Input: part model. Units: mm. Frame: model coordinates. Face numbers are marked on the shaded views. Give positions to 0.01 mm unless a question says otherwise; leave off trailing zeros. Loops run counter-clockwise (first coordinate to the right, second up) from the corner with the lowest first, then second, coordinate; pieces in that order, holes last. Notation, with made-up numbers: M 25,26 L 73,26 A34 ccw 73,59 Z; hole C 61.25,24 d8. An arc over 180 degrees is marked long. Answer as a JSON object with one key per item and string values. Group by question number.
1) Ray query, L1, parallel to Z at x = 0, y = 3.75; L2, parallel to Z at x = 0, y = 6.5. Return the intervals inside material, ascending.
2) Section query B-B on y = 7.25. Return loops of the section in (x, z) (1 decimal), plus the area to 3 significant figures.
3) Draft query along Z for the marked faces 1, 2 and 3. Return one class per face: +Z half, -Z half, draft (parallel to the pull), parting line (faces both ways), or undercut.
4) Section query A-A on z = 0. Return loops of the section in (x, y).
5) Section query C-C on x = 0. Return loops of the section in (y, z).
6) Section query D-D on x = 7.5. Return loops of the section in (y, z).
7) First-contact query: P1, Ø2.5, axis at x = 0, z = 0, coming from the +Y side; P2, Ø6, axis at x = -6, z = 1.5, coming from the -Y side; P3, Ø1.5, axis at x = 5, y = 2, coming from the +Z side; P4, Ø1, axis at y = 6.5, z = -5.5, coming from the +X side. Flat tips, straight axial feed; report the tip coordinate or a pass-through.
Autodesk Inventor part; units mm, degrees
ref_plane "YZ Plane" through (0, 0, 0) normal (1, 0, 0) x (0, 1, 0)
ref_plane "XZ Plane" through (0, 0, 0) normal (0, 1, 0) x (-1, 0, 0)
ref_plane "XY Plane" through (0, 0, 0) normal (0, 0, 1) x (1, 0, 0)
sketch "Sketch1" plane through (0, 0, 0) normal (0, 1, 0) x (-1, 0, 0)
  circle A0 centre (0, 0) radius 13.081
  dimension "outerDiamKnurledKnob" = 26.162
extrude "Extrusion1" add sketch "Sketch1" along normal blind 4.064
sketch "Sketch2" plane through (0, 4.064, 0) normal (0, 1, 0) x (1, 0, 0)
  circle A0 centre (0, 0) radius 7.9375
  dimension "innerRingDiam" = 15.875
extrude "Extrusion2" add sketch "Sketch2" along normal blind 3.937
sketch "Sketch3" plane through (0, 8.001, 0) normal (0, 1, 0) x (1, 0, 0)
  point P0 (0, 0)
  point P1 (0, 0)
hole "Hole1" at (0, 8.001, 0) direction (0, -1, 0) diameter 3.9624 depth 6.35
properties part number "knurledKnob" material "Aluminum 6061"
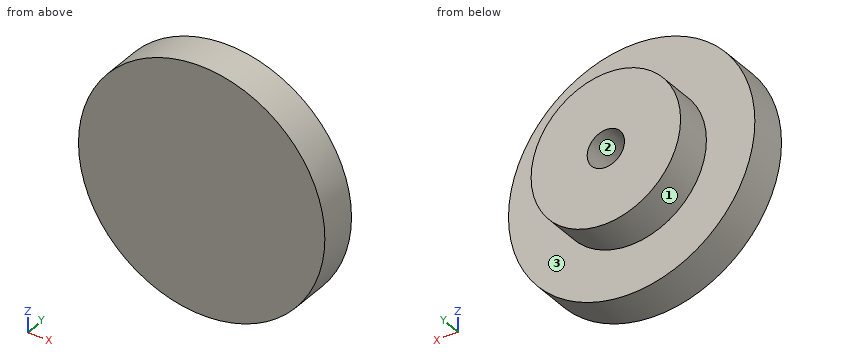
Output:
{
 "1": {"L1": "z = -13.08 to -1.98, 1.98 to 13.08", "L2": "z = -7.94 to -1.98, 1.98 to 7.94"},
 "2": {"outline": "C 0,0 d15.9; hole C 0,0 d4", "area": "186 mm^2"},
 "3": {"face 1": "parting line", "face 2": "undercut", "face 3": "draft"},
 "4": {"outline": "M -13.08,0 L 13.08,0 L 13.08,4.06 L 7.94,4.06 L 7.94,8 L 1.98,8 L 1.98,1.65 L -1.98,1.65 L -1.98,8 L -7.94,8 L -7.94,4.06 L -13.08,4.06 Z"},
 "5": {"outline": "M 0,-13.08 L 4.06,-13.08 L 4.06,-7.94 L 8,-7.94 L 8,-1.98 L 1.65,-1.98 L 1.65,1.98 L 8,1.98 L 8,7.94 L 4.06,7.94 L 4.06,13.08 L 0,13.08 Z"},
 "6": {"outline": "M 0,-10.72 L 4.06,-10.72 L 4.06,-2.6 L 8,-2.6 L 8,2.6 L 4.06,2.6 L 4.06,10.72 L 0,10.72 Z"},
 "7": {"P1": "stops at y = 1.65", "P2": "stops at y = 0", "P3": "stops at z = 12.37", "P4": "stops at x = 6.16"}
}
